```python
from build123d import *

# Parameters (mm, degrees)
SKETCH1_W           = 109.2835
SKETCH1_H           = 61.8236
SKETCH1_R           = 3.46075
SKETCH1_R_2         = 1.6637
SKETCH1_R_3         = 1.524
SKETCH1_R_4         = 1.5875
SKETCH1_W_2         = 50.8
SKETCH1_H_2         = 19.2405
BOSS_EXTRUDE1_DEPTH = 2.54
SKETCH5_W           = 2.54
SKETCH5_H           = 10.4775
SKETCH5_W_2         = 15.9385
SKETCH5_H_2         = 3.429
CUT_EXTRUDE1_DEPTH  = 1.905
FILLET1_R           = 1.27
FILLET2_R           = 2.54
SKETCH6_R           = 1.6637
BOSS_EXTRUDE2_DEPTH = 2.54
SKETCH7_R           = 1.3335
BOSS_EXTRUDE3_DEPTH = 3.81


with BuildPart() as part:
    # Sketch1 → Boss-Extrude1 (new body)
    with BuildSketch(Plane(origin=(0, 0, 0), x_dir=(1, 0, 0), z_dir=(0, 1, 0))):
        with Locations((19.08175, 0)):
            Rectangle(SKETCH1_W, SKETCH1_H)
        with Locations(Location((44.1325, 14.8209, 0), (0, 0, 270))):
            Circle(SKETCH1_R, mode=Mode.SUBTRACT)
        with Locations(Location((-30.02, 25.8718, 0), (0, 0, 270))):
            Circle(SKETCH1_R_2, mode=Mode.SUBTRACT)
        with Locations(Location((30.02, 25.8718, 0), (0, 0, 90))):
            Circle(SKETCH1_R_2, mode=Mode.SUBTRACT)
        with Locations(Location((-30.02, 3.77, 0), (0, 0, 90))):
            Circle(SKETCH1_R_2, mode=Mode.SUBTRACT)
        with Locations(Location((30.02, 3.77, 0), (0, 0, 270))):
            Circle(SKETCH1_R_2, mode=Mode.SUBTRACT)
        with Locations(Location((30.02, -3.77, 0), (0, 0, 90))):
            Circle(SKETCH1_R_2, mode=Mode.SUBTRACT)
        with Locations(Location((-30.02, -3.77, 0), (0, 0, 270))):
            Circle(SKETCH1_R_2, mode=Mode.SUBTRACT)
        with Locations(Location((-30.02, -25.8718, 0), (0, 0, 90))):
            Circle(SKETCH1_R_2, mode=Mode.SUBTRACT)
        with Locations(Location((30.02, -25.8718, 0), (0, 0, 270))):
            Circle(SKETCH1_R_2, mode=Mode.SUBTRACT)
        with Locations(Location((63.21425, 0, 0), (0, 0, 270))):
            Circle(SKETCH1_R_3, mode=Mode.SUBTRACT)
        with Locations(Location((69.9135, 27.1018, 0), (0, 0, 270))):
            Circle(SKETCH1_R_4, mode=Mode.SUBTRACT)
        with Locations(Location((69.9135, -27.1018, 0), (0, 0, 270))):
            Circle(SKETCH1_R_4, mode=Mode.SUBTRACT)
        with Locations((-1.32, 14.8209)):
            Rectangle(SKETCH1_W_2, SKETCH1_H_2, mode=Mode.SUBTRACT)
        with Locations((-1.32, -14.8209)):
            Rectangle(SKETCH1_W_2, SKETCH1_H_2, mode=Mode.SUBTRACT)
    extrude(amount=BOSS_EXTRUDE1_DEPTH)

    # Sketch5 → Cut-Extrude1 (cut)
    with BuildSketch(Plane.XZ):
        with Locations((27.255, -14.8209)):
            Rectangle(SKETCH5_W, SKETCH5_H)
        with Locations((27.255, 14.8209)):
            Rectangle(SKETCH5_W, SKETCH5_H)
        with Locations((63.21425, 14.351)):
            Rectangle(SKETCH5_W_2, SKETCH5_H_2)
    extrude(amount=-CUT_EXTRUDE1_DEPTH, mode=Mode.SUBTRACT)

    # Fillet1
    fillet1_edges = [part.edges().sort_by_distance(p)[0] for p in [
        (25.985, 1.905, -14.8209),
        (27.255, 1.905, -9.58215),
        (28.525, 1.905, -14.8209),
        (27.255, 1.905, -20.05965),
        (25.985, 1.905, 14.8209),
        (27.255, 1.905, 20.05965),
        (28.525, 1.905, 14.8209),
        (27.255, 1.905, 9.58215),
        (71.1835, 1.905, 14.351),
        (71.1835, 0.9525, 16.0655),
        (63.21425, 1.905, 12.6365),
        (71.1835, 0.9525, 12.6365),
        (55.245, 1.905, 14.351),
        (55.245, 0.9525, 12.6365),
        (63.21425, 1.905, 16.0655),
        (55.245, 0.9525, 16.0655),
    ]]
    fillet(fillet1_edges, radius=FILLET1_R - 0.0001)  # a hair under: the kernel refuses the full size

    # Fillet2
    fillet2_edges = [part.edges().sort_by_distance(p)[0] for p in [
        (-35.56, 1.27, -30.9118),
        (73.7235, 1.27, -30.9118),
        (73.7235, 1.27, 30.9118),
        (-35.56, 1.27, 30.9118),
    ]]
    fillet(fillet2_edges, radius=FILLET2_R)

    # Sketch6 → Boss-Extrude2 (add)
    with BuildSketch(Plane.XZ):
        with Locations((-30.02, 3.77)):
            Circle(SKETCH6_R)
        with Locations((-30.02, -3.77)):
            Circle(SKETCH6_R)
        with Locations((30.02, -25.8718)):
            Circle(SKETCH6_R)
        with Locations((30.02, 25.8718)):
            Circle(SKETCH6_R)
        with Locations((30.02, 3.77)):
            Circle(SKETCH6_R)
        with Locations((30.02, -3.77)):
            Circle(SKETCH6_R)
    extrude(amount=-BOSS_EXTRUDE2_DEPTH)

    # Sketch7 → Boss-Extrude3 (add)
    with BuildSketch(Plane.XZ):
        with Locations(Location((-30.02, 3.77, 0), (0, 0, 90))):
            Circle(SKETCH7_R)
        with Locations(Location((-30.02, -3.77, 0), (0, 0, 90))):
            Circle(SKETCH7_R)
        with Locations(Location((30.02, -25.8718, 0), (0, 0, 90))):
            Circle(SKETCH7_R)
        with Locations(Location((30.02, 25.8718, 0), (0, 0, 90))):
            Circle(SKETCH7_R)
        with Locations(Location((30.02, -3.77, 0), (0, 0, 90))):
            Circle(SKETCH7_R)
        with Locations(Location((30.02, 3.77, 0), (0, 0, 90))):
            Circle(SKETCH7_R)
    extrude(amount=BOSS_EXTRUDE3_DEPTH)


solid = part.part
```
Input: part model. Units: mm. Frame: model coordinates. A direction names the side the tool comes from. Give positions to 0.01 mm unless a question says otherwise; leave off trailing zeros. Order: outer loops, then holes, each group sorted by start corner. A loop starts at its lowest first (then second) coordinate and runs counter-clockwise, first axis right, second up. Notation, with made-up numbers: M 21,12 L 60,12 A23 cw 60,34 Z; hole C 81,52.25 d4. An arc over 180 degrees is marked long. One line per question, with ' | ' between items.
1) Contact query for flat-ended pins moving along their axis: P1, Ø10, axis at x = 57.5, z = 2, coming from the -Y side; P2, Ø0.7, axis at x = 62.5, z = 14.5, coming from the -Y side; P3, Ø3, axis at x = 35, y = -0.5, coming from the -Z side. Output: stop coordinate, or through.
Filled in:
P1: stops at y = 0 | P2: stops at y = 1.9 | P3: stops at z = -30.91
2) Section A-A on y = -2.25. Output: boundary loops of the cut face in (x, z).
Filled in:
outline: C -30.02,-3.77 d2.67; C -30.02,3.77 d2.67; C 30.02,-25.87 d2.67; C 30.02,-3.77 d2.67; C 30.02,3.77 d2.67; C 30.02,25.87 d2.67
3) Section C-C on x = 22.5. Output: boundary loops of the cut face in (y, z).
Filled in:
outline: M 0,-30.91 L 2.54,-30.91 L 2.54,-24.44 L 0,-24.44 Z; M 0,-5.2 L 2.54,-5.2 L 2.54,5.2 L 0,5.2 Z; M 0,24.44 L 2.54,24.44 L 2.54,30.91 L 0,30.91 Z
4) Access query for faces 1 (the face through (18, 1, 30.912)), 2 (the face through (-2, 1, -5.201)), 3 (the face through (28.896, -1.878, 26.589)). Directions: +Z, -Z, +X, -X, +Y, -Y. A direction counts if a zero-diameter tool reaches every point of the face in a straight line with its end or side. Return the directions, or none.
Filled in:
face 1: +Z, +X, -X, +Y, -Y | face 2: +Y, -Y | face 3: -Y
5) Section D-D on z = -13.5. State how many separate pieces and enclosed holes the cut face has, and give its area (3 significant figures).
Filled in:
separate pieces: 3 | enclosed holes: 0 | area: 128 mm2
6) Section B-B on z = -22. Output: boundary loops of the cut face in (x, y), and give its area (3 significant figures).
Filled in:
outline: M -35.56,0 L -26.72,0 L -26.72,2.54 L -35.56,2.54 Z; M 24.08,0 L 73.72,0 L 73.72,2.54 L 24.08,2.54 Z | area: 149 mm2
7) Ray query, L1, parallel to Z at x = -14.5, y = 1.25; L2, parallel to X at y = 0.25, z = -20.5; L3, parallel to X at y = 1.25, z = -18. Return the intervals inside material, ascending.
Filled in:
L1: z = -30.91 to -24.44, -5.2 to 5.2, 24.44 to 30.91 | L2: x = -35.56 to -26.72, 24.08 to 73.72 | L3: x = -35.56 to -26.72, 24.08 to 26.14, 28.37 to 42.76, 45.5 to 73.72
8) Draft query along X for faces 4 (the face through (29.62, -1.88, -24.6)), 5 (the face through (-30, -3.81, 4)), 6 (the face through (-28.84, -1.88, 4.39)). Return one class per face: pulls with the +X half, pulls with the -X half, needs draft (parallel to the pull), parting line crosses it, or undercut.
Filled in:
face 4: parting line crosses it | face 5: needs draft | face 6: undercut
